For this review, take the finished solid that the model builds, in its own axes (mm). A direction names the side the tool comes from. Round coordinates to 2 decimals unless told otherwise and drop trailing zeros. Write each loop counter-clockwise with the first axis right and the second up, starting at its lowest first coordinate (ties: lowest second). Pieces come first, ordered by that corner, then holes. Notation, with made-up numbers: M -21,-36 L 3,-36 A29 ccw 3,-7 Z; hole C 68.5,23 d7. An arc over 180 degrees is marked long. Write each question's results on one line, items separated by ' | '. Start each with the question number.
```python
from build123d import *

# Parameters (mm, degrees)
SKETCH1_R           = 1.7
BOSS_EXTRUDE1_DEPTH = 6
BOSS_EXTRUDE2_START = 6
BOSS_EXTRUDE2_DEPTH = 6
SKETCH2_R           = 3.1
CUT_EXTRUDE1_DEPTH  = 3
FILLET1_R           = 2
FILLET2_R           = 6
FILLET3_R           = 1
FILLET4_R           = 1
FILLET5_DEPTH       = 6
FILLET5_START       = -1
FILLET5_3_DEPTH     = 13
FILLET5_START_2     = 6.9999999
FILLET5_4_DEPTH     = 5.0000001
FILLET5_5_DEPTH     = 6


with BuildPart() as part:
    # Sketch1 → Boss-Extrude1 (new body)
    with BuildSketch(Plane.XY):
        with BuildLine():
            Line((4, 0), (150.292108611, 0))
            Line((150.292108611, 0), (176.628985356, 43.386559906))
            ThreePointArc((176.628985356, 43.386559906), (176.393105018, 49.97239446), (170.254392606, 52.369281235))
            Line((170.254392606, 52.369281235), (151.015607145, 48.286332665))
            ThreePointArc((151.015607145, 48.286332665), (149.926554244, 48.177660945), (148.839947189, 48.308545892))
            Line((148.839947189, 48.308545892), (139.910123035, 50.395083576))
            ThreePointArc((139.910123035, 50.395083576), (136.514088914, 49.633727185), (135, 46.5))
            Line((135, 46.5), (135, 39))
            Line((135, 39), (111, 39))
            Line((111, 39), (105, 45))
            Line((105, 45), (14, 45))
            Line((14, 45), (14, 122))
            Line((14, 122), (18.5, 122))
            ThreePointArc((18.5, 122), (22.5, 126), (18.5, 130))
            Line((18.5, 130), (4, 130))
            Line((4, 130), (4, 0))
        make_face()
        with BuildLine():
            Line((33.15, 5.69), (37.15, 5.69))
            ThreePointArc((37.15, 5.69), (38.95, 3.89), (37.15, 2.09))
            Line((37.15, 2.09), (33.15, 2.09))
            ThreePointArc((33.15, 2.09), (31.35, 3.89), (33.15, 5.69))
        make_face(mode=Mode.SUBTRACT)
        with Locations((115.15, 3.89)):
            Circle(SKETCH1_R, mode=Mode.SUBTRACT)
        with Locations((171.5, 46.5)):
            Circle(SKETCH1_R, mode=Mode.SUBTRACT)
        with Locations((18.5, 126)):
            Circle(SKETCH1_R, mode=Mode.SUBTRACT)
        with Locations((139, 46.5)):
            Circle(SKETCH1_R, mode=Mode.SUBTRACT)
    extrude(amount=BOSS_EXTRUDE1_DEPTH)

    # Sketch1<3> → Boss-Extrude2 (add)
    with BuildSketch(Plane.XY.offset(BOSS_EXTRUDE2_START)):
        with BuildLine():
            Line((12, 33.156912913), (29.769570295, 6.545367431))
            ThreePointArc((29.769570295, 6.545367431), (31.818094908, 8.879830504), (34.759400799, 9.877272523))
            Line((34.759400799, 9.877272523), (12, 43.961542399))
            Line((12, 43.961542399), (12, 130))
            Line((12, 130), (6, 130))
            Line((6, 130), (6, 0))
            Line((6, 0), (12, 0))
            Line((12, 0), (12, 33.156912913))
        make_face()
        with BuildLine():
            ThreePointArc((117.028697802, 9.58828874), (119.626144393, 7.885513906), (121.024211708, 5.112144348))
            Line((121.024211708, 5.112144348), (144.292108611, 25.881627522))
            Line((144.292108611, 25.881627522), (144.292108611, 0))
            Line((144.292108611, 0), (150.292108611, 0))
            Line((150.292108611, 0), (150.292108611, 31.237371514))
            Line((150.292108611, 31.237371514), (159.087870064, 39.088679274))
            Line((159.087870064, 39.088679274), (150.077765021, 39.088679274))
            Line((150.077765021, 39.088679274), (117.028697802, 9.58828874))
        make_face()
    extrude(amount=BOSS_EXTRUDE2_DEPTH)

    # Sketch2 → Cut-Extrude1 (cut)
    with BuildSketch(Plane(origin=(0, 0, 0), x_dir=(-1, 0, 0), z_dir=(0, 0, -1))):
        with Locations((-139, 46.5)):
            Circle(SKETCH2_R)
    extrude(amount=-CUT_EXTRUDE1_DEPTH, mode=Mode.SUBTRACT)

    # Fillet1
    fillet1_edges = [part.edges().sort_by_distance(p)[0] for p in [
        (150.077765021, 39.088679274, 9),
        (117.028697802, 9.58828874, 9),
        (121.024211708, 5.112144348, 9),
        (144.292108611, 25.881627522, 9),
        (12, 33.156912913, 9),
        (29.769570295, 6.545367431, 9),
        (34.759400799, 9.877272523, 9),
    ]]
    fillet(fillet1_edges, radius=FILLET1_R)

    # Fillet2
    fillet2_edges = [part.edges().sort_by_distance(p)[0] for p in [
        (150.292108611, 31.237371514, 9),
        (12, 43.961542399, 9),
    ]]
    fillet(fillet2_edges, radius=FILLET2_R)

    # Fillet3
    fillet3_edges = [part.edges().sort_by_distance(p)[0] for p in [
        (159.087870064, 39.088679274, 9),
    ]]
    fillet(fillet3_edges, radius=FILLET3_R)

    # Fillet4
    fillet4_edges = [part.edges().sort_by_distance(p)[0] for p in [
        (150.292108611, 14.275239757, 6),
        (144.292108611, 10.70775043, 6),
        (31.818094908, 8.879830504, 6),
        (21.955332725, 18.24789794, 6),
        (132.014705022, 14.922522436, 6),
        (119.626144393, 7.885513906, 6),
        (134.291167915, 24.997183839, 6),
        (143.109520399, 23.24083315, 6),
        (13.419721476, 28.474156966, 6),
        (29.643487506, 7.953534135, 6),
        (33.507072774, 10.53340121, 6),
        (121.499193347, 6.443768461, 6),
        (118.405499352, 9.909610742, 6),
        (150.127840882, 38.957381532, 6),
        (23.123694308, 27.302799836, 6),
        (150.816111741, 31.002714877, 6),
        (12.258093391, 44.039791347, 6),
        (153.653220831, 39.088679274, 6),
        (154.714203524, 35.184639557, 6),
        (157.400244487, 38.445032985, 6),
        (12, 13.280094048, 6),
        (12, 87.89031346, 6),
        (6, 65, 6),
    ]]
    fillet(fillet4_edges, radius=FILLET4_R)

    # Fillet5: read off the stored shape, not the designer's step
    # Fillet5 outline → Fillet5 (add)
    with BuildSketch(Plane.XY):
        with BuildLine():
            ThreePointArc((135, 42), (134.121320344, 39.878679656), (132, 39))
            Line((132, 39), (135, 39))
            Line((135, 39), (135, 42))
        make_face()
        with BuildLine():
            ThreePointArc((112.242640687, 39), (111.09459039, 39.228361402), (110.121320344, 39.878679656))
            Line((110.121320344, 39.878679656), (111, 39))
            Line((111, 39), (112.242640687, 39))
        make_face()
    extrude(amount=FILLET5_DEPTH)

    # Fillet5 2 outline → Fillet5 2 (revolve, cut)
    with BuildSketch(Plane(origin=(151.292108611, 0, 7), x_dir=(1, 0, 0), z_dir=(0, 0, 1))):
        with BuildLine():
            ThreePointArc((4, 0), (1.878679656, 0.878679656), (1, 3))
            Line((1, 3), (1, 0))
            Line((1, 0), (4, 0))
        make_face()
    revolve(axis=Axis((151.292108611, 0, 7), (0, 1, 0)), mode=Mode.SUBTRACT)

    # Fillet5 3 outline → Fillet5 3 (cut)
    with BuildSketch(Plane.XY.offset(FILLET5_START)):
        with BuildLine():
            Line((150.292108611, 0), (151.168220622, 1.443279953))
            ThreePointArc((151.168220622, 1.443279953), (150.075094632, 0.385601394), (148.603727944, 0))
            Line((148.603727944, 0), (150.292108611, 0))
        make_face()
        with BuildLine():
            ThreePointArc((7, 0), (4.878679656, 0.878679656), (4, 3))
            Line((4, 3), (4, 0))
            Line((4, 0), (7, 0))
        make_face()
        with BuildLine():
            Line((7, 130), (4, 130))
            Line((4, 130), (4, 127))
            ThreePointArc((4, 127), (4.878679656, 129.121320344), (7, 130))
        make_face()
        with BuildLine():
            Line((105, 45), (103.757359313, 45))
            ThreePointArc((103.757359313, 45), (104.90540961, 44.771638598), (105.878679656, 44.121320344))
            Line((105.878679656, 44.121320344), (105, 45))
        make_face()
    extrude(amount=FILLET5_3_DEPTH, mode=Mode.SUBTRACT)

    # Fillet5 4 outline → Fillet5 4 (cut)
    with BuildSketch(Plane.XY.offset(FILLET5_START_2)):
        with BuildLine():
            ThreePointArc((148.603727944, 0), (149.487080244, 0.13300005), (150.292108611, 0.520207524))
            Line((150.292108611, 0.520207524), (150.292108611, 3))
            ThreePointArc((150.292108611, 3), (149.413428955, 0.878679656), (147.292108611, 0))
            Line((147.292108611, 0), (148.603727944, 0))
        make_face()
    extrude(amount=FILLET5_4_DEPTH, mode=Mode.SUBTRACT)

    # Fillet5 5 outline → Fillet5 5 (add)
    with BuildSketch(Plane.XY):
        with BuildLine():
            ThreePointArc((17, 45), (14.878679656, 45.878679656), (14, 48))
            Line((14, 48), (14, 45))
            Line((14, 45), (17, 45))
        make_face()
        with BuildLine():
            ThreePointArc((14, 119), (14.878679656, 121.121320344), (17, 122))
            Line((17, 122), (14, 122))
            Line((14, 122), (14, 119))
        make_face()
    extrude(amount=FILLET5_5_DEPTH)


solid = part.part
```
Item 1: We need section B-B on x = 93. State the section outline as (y, z) points.
Item 2: We need section A-A on y = 100.5. State the section outline as (x, z) points.
Item 3: Mouldability with a two-part tool opening along Y and no side actions: class faces 1 (the flat face through (12, 13, 9)), 2 (the cylindrical face through (19.3, 124.5, 3)), 3 (the cylindrical face through (150.83, 31.03, 9.54)) as pulls with the +Y half, pulls with the -Y half, needs draft (parallel to the pull), parting line crosses it, or undercut.
Item 4: Insertion check: P1, Ø6, axis at y = 71, z = 7.5, coming from the +X side; P2, Ø8, axis at x = 139, y = 46.5, coming from the +Z side; P3, Ø3, axis at x = 118.5, z = 4.5, coming from the +Y side. Each pin has a flat end and moves straight along its axis. Give the tip position at first contact, or say it passes through.
Item 5: For probe 1 along Y at (x, z) = (139, 4.3); probe 2 along Y at (x, z) = (47.5, 5.75); probe 3 along X at (y, z) = (57, 4.25), list the stretches that pass through material, from the lowest coordinate up.
Item 6: For faces 4 (the flat face through (21.867, 18.38, 9.465)), 5 (the flat face through (150.292, 16, 9)), 6 (the cylindrical face through (133.88, 25.03, 6.29)), 7 (the flat face through (12, 87, 9)), list the 3-axis set-ups (+Z, -Z, +X, -X, +Y, -Y) from which the entire face can be reached by the end or side of a thin tool; tool diameter is ignored.
Numbers:
1) outline: M 0,0 L 45,0 L 45,6 L 0,6 Z
2) outline: M 4,0 L 14,0 L 14,6 L 13,6 A1 cw 12,7 L 12,12 L 6,12 L 6,7 A1 cw 5,6 L 4,6 Z
3) face 1: needs draft | face 2: undercut | face 3: pulls with the -Y half
4) P1: stops at x = 14 | P2: stops at z = 6 | P3: stops at y = 39
5) probe 1: y = 0 to 44.8, 48.2 to 50.5 | probe 2: y = 0 to 45 | probe 3: x = 4 to 14
6) face 4: +Z, -Y | face 5: +Z, +X, -Y | face 6: +Z, +Y | face 7: +Z, +X, +Y
